Build history of the part. All positions in model axes, mm. A direction names the side the tool comes from. Give positions to 0.01 mm unless a question says otherwise; leave off trailing zeros. Loops run counter-clockwise (first coordinate to the right, second up) from the corner with the lowest first, then second, coordinate; pieces in that order, holes last. Notation, with made-up numbers: M 87,31.25 L 137,31.25 A17 ccw 137,50.25 Z; hole C 28.25,-12 d2. An arc over 180 degrees is marked long. Put each result on its own line as item: value.
Autodesk Inventor part; units mm, degrees
ref_plane "Work Plane2" through (0, 12, 0) normal (0, 1, 0) x (1, 0, 0)
ref_plane "Work Plane1" through (0, -10, 0) normal (0, -1, 0) x (1, 0, 0)
ref_plane "YZ Plane" through (0, 0, 0) normal (1, 0, 0) x (0, 1, 0)
sketch "Sketch1" plane through (0, 0, 0) normal (0, 1, 0) x (-1, 0, 0)
  line L0 (-17.6, 17.6) -> (17.6, 17.6)
  line L1 (17.6, 17.6) -> (17.6, -17.6)
  line L2 (17.6, -17.6) -> (-17.6, -17.6)
  line L3 (-17.6, -17.6) -> (-17.6, 17.6)
  line L4 (-17.6, 17.6) -> (17.6, -17.6) construction
  line L5 (17.6, 17.6) -> (-17.6, -17.6) construction
  point P0 (0, 0)
  dimension "d0" = 35.2
  dimension "d1" = 35.2
extrude "Extrusion1" add sketch "Sketch1" along normal mid plane 36
sketch "Sketch2" plane through (0, 18, 0) normal (0, 1, 0) x (1, 0, 0)
  circle A0 centre (0, 0) radius 11
  dimension "d4" = 22
extrude "Extrusion2" add sketch "Sketch2" along normal blind 2
sketch "Sketch3" plane through (0, 18, 0) normal (0, 1, 0) x (1, 0, 0)
  circle A0 centre (0, 0) radius 2.5
  dimension "d7" = 5
extrude "Extrusion3" add sketch "Sketch3" along normal blind 24
sketch "Sketch4" plane through (0, 42, 0) normal (0, 1, 0) x (1, 0, 0)
  circle A0 centre (0, 0) radius 2.5
  line L0 (-2, -1.5) -> (-2, 1.5)
  circle A1 centre (0, 0) radius 2.5
  dimension "d10" = 4.5
extrude "Extrusion4" cut sketch "Sketch4" against normal blind 15 contours L0 A0 picked at (-2.0912, -0.3466)
ref_plane "Work Plane2" through (0, 12, 0) normal (0, 1, 0) x (1, 0, 0)
ref_plane "Work Plane1" through (0, -10, 0) normal (0, -1, 0) x (1, 0, 0)
sketch "Sketch5" plane through (0, -10, 0) normal (0, -1, 0) x (1, 0, 0)
  line L0 (-17.6, -17.6) -> (17.6, -17.6)
  line L1 (17.6, -17.6) -> (17.6, 17.6)
  line L2 (17.6, 17.6) -> (-17.6, 17.6)
  line L3 (-17.6, 17.6) -> (-17.6, -17.6)
  line L4 (-17.59, -17.59) -> (17.59, -17.59)
  line L5 (17.59, -17.59) -> (17.59, 17.59)
  line L6 (17.59, 17.59) -> (-17.59, 17.59)
  line L7 (-17.59, 17.59) -> (-17.59, -17.59)
  point P0 (0, 0)
  dimension "d14" = 0.01
extrude "Extrusion5" cut sketch "Sketch5" against normal up to surface (22 mm away)
chamfer "Chamfer1" distance 4 angle 45 4 edges at (-17.59, 1, 17.59) (-17.59, 1, -17.59) (17.59, 1, 17.59) (17.59, 1, -17.59)
chamfer "Chamfer2" distance 2 angle 45 8 edges at (-17.6, 15, 17.6) (-17.6, -14, 17.6) (17.6, 15, 17.6) (17.6, -14, 17.6) (-17.6, -14, -17.6) (17.6, 15, -17.6) (17.6, -14, -17.6) (-17.6, 15, -17.6)
sketch "Sketch6" plane through (0, -18, 0) normal (0, -1, 0) x (1, 0, 0)
  circle A0 centre (0, 0) radius 2.5
  circle A1 centre (0, 0) radius 2.5
  dimension "d24" = 5
extrude "Extrusion6" add sketch "Sketch6" along normal blind 13
fillet "Fillet1" radius 1 1 edges at (-2.5, -31, 0)
sketch "Sketch7" plane through (0, -18, 0) normal (0, -1, 0) x (1, 0, 0)
  circle A0 centre (0, 0) radius 1.5
  circle A1 centre (0, 0) radius 9.525
  point P0 (-9.525, 0)
  point P1 (9.525, 0)
  dimension "d28" = 19.05
hole "Hole1" at (-9.525, -18, 0) at (9.525, -18, 0) direction (0, 1, 0) diameter 2.013 depth 7.6 tip angle 118
properties part number "NEMA_14_Dual_LM1048"
Q1. Probe line 1 (X direction, y = -13.75, z = 0); line 2 (Z direction, x = 3, y = 10.5). List the from-to ranges inside material, lowest first. Write a range as from..to.
Here are the results:
line 1: -17.6..-10.53, -8.52..8.52, 10.53..17.6
line 2: -17.59..17.59
Q2. Slice it at B-B (y = -8.5). List the corners of the cut face in (x, z).
Here are the results:
outline: M -17.59,-13.59 L -13.59,-17.59 L 13.59,-17.59 L 17.59,-13.59 L 17.59,13.59 L 13.59,17.59 L -13.59,17.59 L -17.59,13.59 Z
Q3. Drop flat-ended pins along their axis: pin 1 Ø12 at (x, z) = (-10, -7) entering from -Y; pin 2 Ø1.5 at (y, z) = (32.5, -0.5) entering from -X; pin 3 Ø17.5 at (y, z) = (-1, 2.5) entering from -X. Give the stop position or say it passes through.
Here are the results:
pin 1: y = -18
pin 2: x = -2
pin 3: x = -17.59
Q4. Mould opens along Y. For faces 5 (the flat face through (0, 42, 0)), 6 (the flat face through (15.62, 0.85, -15.56)), 7 (the flat face through (0, -14, 17.6)) say: pulls with the +Y half, pulls with the -Y half, needs draft (parallel to the pull), parting line crosses it, or undercut.
Here are the results:
face 5: pulls with the +Y half
face 6: undercut
face 7: needs draft
Q5. Tool access for faces 1 (the flat face through (-2, 35, 0)), 2 (the conical face through (9.37, -9.9, -0.08)), 3 (the flat face through (15.56, 0.85, 15.62)), 4 (the cylindrical face through (-2.38, 18.99, -10.74)): list every direction of +Z, -Z, +X, -X, +Y, -Y with a clear straight run to the whole face (end or side of a thin tool).
Here are the results:
face 1: +Z, -Z, -X, +Y
face 2: -Y
face 3: +Z, +X
face 4: +Y
